Geometry: final body of the model. Coordinates: model frame, mm. Face numbers are marked on the shaded views. A direction names the side the tool comes from. Give positions to 0.01 mm unless a question says otherwise; leave off trailing zeros. Write each loop counter-clockwise with the first axis right and the second up, starting at its lowest first coordinate (ties: lowest second). Pieces come first, ordered by that corner, then holes. Notation, with made-up numbers: (2, 70.25) -> (49, 70.25) arc R14 ccw to (49, 74.25) -> close; hole circle Ø10 at (50, 22). An arc over 180 degrees is marked (long way). Answer as a JSON object with one key per item and string values. Group by question number.
(1) Section query B-B on z = 11.5. Output: boundary loops of the cut face in (x, y), plus the area to 3 significant figures.
(2) Set-up query: the marked faces 4 and 5. Return all of +Z, -Z, +X, -X, +Y, -Y with unobstructed straight access to the full face (end or side cutting, diameter ignored); none if empty.
(3) Material intervals for probe 1 along Y at (x, z) = (12, 52); probe 2 along X at (y, z) = (-10.5, 36); probe 3 along Z at (x, y) = (-11.2, 17), sorted ascending.
(4) Contact query for flat-ended pins moving along their axis: pin 1 Ø7 at (y, z) = (17, 52) entering from +X; pin 2 Ø2 at (x, z) = (-11, 23.5) entering from +Y; pin 3 Ø1 at (x, y) = (-12, 9) entering from -Z; pin 4 Ø3 at (x, z) = (3.5, 48) entering from +Y. Output: stop coordinate, or through.
(5) Draft query along X for the marked faces 1, 2 and 3. Return one class per face: +X half, -X half, draft (parallel to the pull), parting line (faces both ways), or undercut.
(6) Section query D-D on x = -0.25. Output: boundary loops of the cut face in (y, z), plus the area to 3 significant figures.
(7) Section query A-A on y = 4. Output: boundary loops of the cut face in (x, z), plus the area to 3 significant figures.
(8) Section query C-C on y = -3. Output: boundary loops of the cut face in (x, z).
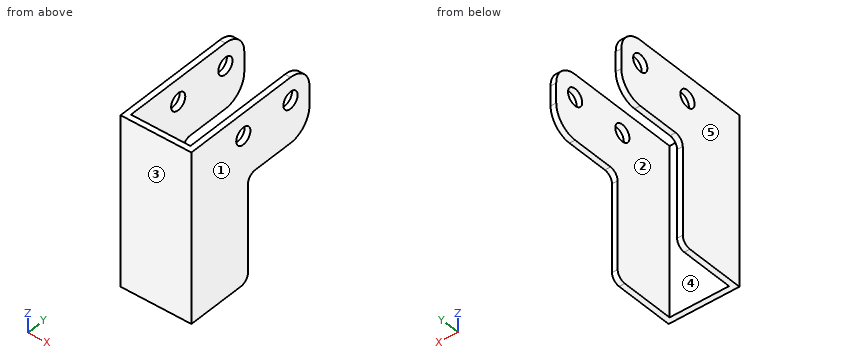
Autodesk Inventor part; units mm, degrees
ref_plane "YZ Plane" through (0, 0, 0) normal (1, 0, 0) x (0, 1, 0)
ref_plane "XZ Plane" through (0, 0, 0) normal (0, 1, 0) x (-1, 0, 0)
ref_plane "XY Plane" through (0, 0, 0) normal (0, 0, 1) x (1, 0, 0)
sketch "スケッチ1" plane through (0, 0, 0) normal (0, 0, 1) x (1, 0, 0)
  line L0 (-12.5, 25) -> (12.5, 25)
  line L1 (12.5, 25) -> (12.5, -25)
  line L2 (12.5, -25) -> (-12.5, -25)
  line L3 (-12.5, -25) -> (-12.5, 25)
  line L4 (-10.5, 25) -> (10.5, 25)
  line L5 (10.5, 25) -> (10.5, -23)
  line L6 (10.5, -23) -> (-10.5, -23)
  line L7 (-10.5, -23) -> (-10.5, 25)
  point P0 (0, 0)
  dimension "d0" = 25
  dimension "d1" = 50
  dimension "d2" = 25
  dimension "d3" = 12.5
  dimension "d4" = 2
  dimension "d5" = 2
  dimension "d6" = 2
extrude "押し出し1" add sketch "スケッチ1" along normal blind 60 contours L0 L7 L6 L5 L1 L2 L3
sketch "スケッチ2" plane through (12.5, -25, 0) normal (1, 0, 0) x (0, 0, -1)
  line L0 (0, 50) -> (-60, 50)
  line L1 (-30, 50) -> (-30, 0)
  line L2 (0, 0) -> (-60, 0)
  line L3 (-60, 50) -> (-60, 0)
  point P0 (0, 25)
  point P1 (-52, 42)
  point P2 (-52, 22)
  dimension "d12" = 8
  dimension "d76" = 8
  dimension "d85" = 8
  dimension "d86" = 20
hole "Hole1" at (12.5, 17, 52) at (12.5, -3, 52) direction (-1, 0, 0) diameter 6 end through all
sketch "スケッチ9" plane through (12.5, -25, 0) normal (1, 0, 0) x (0, 0, -1)
  circle A0 centre (-52, 22) radius 3
  line L0 (0, 50) -> (-37, 50)
  line L1 (-37, 50) -> (-37, 24)
  line L2 (-37, 24) -> (0, 24)
  line L3 (0, 24) -> (0, 50)
  line L4 (0, 2) -> (-60, 2)
  point P0 (0, 25)
  dimension "d77" = 15
  dimension "d78" = 22
extrude "押し出し5" cut sketch "スケッチ9" against normal through all contours L3 L2 L1 L0
fillet "フィレット5" radius 3 2 edges at (11.5, -1, 37) (-11.5, -1, 37)
fillet "フィレット6" radius 8 4 edges at (-11.5, 25, 60) (11.5, 25, 60) (11.5, 25, 37) (-11.5, 25, 37)
fillet "フィレット7" radius 3 2 edges at (11.5, -1, 0) (-11.5, -1, 0)
equation "\"d1\" = 2 * d0"
equation "\"d4\" = d5"
equation "\"d6\" = d5"
properties part number "CounterWeight" material "アルミニウム 6061"
Answer list:
{
 "1": {"outline": "(-12.5, -25) -> (12.5, -25) -> (12.5, -1) -> (10.5, -1) -> (10.5, -23) -> (-10.5, -23) -> (-10.5, -1) -> (-12.5, -1) -> close", "area": "138 mm2"},
 "2": {"face 4": "+Z, -Z, +Y", "face 5": "+Z, -Z, -X, +Y, -Y"},
 "3": {"probe 1": "-25 to -6, 0 to 14, 20 to 25", "probe 2": "-12.5 to -10.5, 10.5 to 12.5", "probe 3": "37 to 49, 55 to 60"},
 "4": {"pin 1": "x = 12.5", "pin 2": "y = -1", "pin 3": "z = 37", "pin 4": "y = -23"},
 "5": {"face 1": "+X half", "face 2": "undercut", "face 3": "draft"},
 "6": {"outline": "(-25, 0) -> (-23, 0) -> (-23, 60) -> (-25, 60) -> close", "area": "120 mm2"},
 "7": {"outline": "(-12.5, 37) -> (-10.5, 37) -> (-10.5, 60) -> (-12.5, 60) -> close; (10.5, 37) -> (12.5, 37) -> (12.5, 60) -> (10.5, 60) -> close", "area": "92.0 mm2"},
 "8": {"outline": "(-12.5, 0.17) -> (-10.5, 0.17) -> (-10.5, 49) -> (-12.5, 49) -> close; (-12.5, 55) -> (-10.5, 55) -> (-10.5, 60) -> (-12.5, 60) -> close; (10.5, 0.17) -> (12.5, 0.17) -> (12.5, 49) -> (10.5, 49) -> close; (10.5, 55) -> (12.5, 55) -> (12.5, 60) -> (10.5, 60) -> close"}
}
